Verification items for the finished model (mm, model axes). Face numbers are marked on the shaded views. Coordinates: 2 decimals unless noted, no trailing zeros. Loops run counter-clockwise (first coordinate to the right, second up) from the corner with the lowest first, then second, coordinate; pieces in that order, holes last. Notation, with made-up numbers: (4, -29.75) -> (19, -29.75) arc R28 ccw to (19, 4.25) -> close; hole circle Ø1 at (26, 39). An arc over 180 degrees is marked (long way). Use CSV: the item, a comma, the result in double quotes. Start each with the question number.
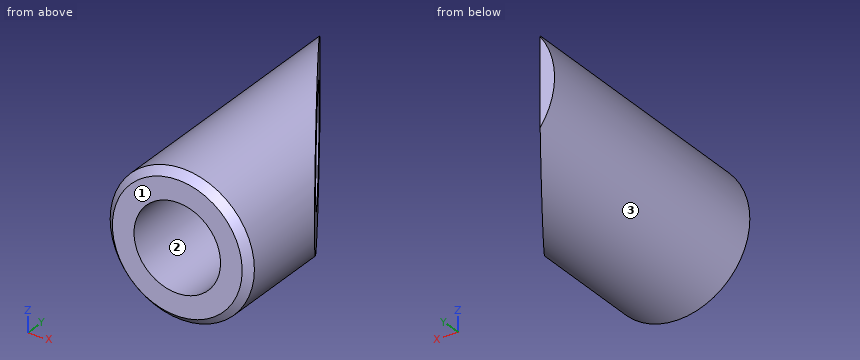
```python
from build123d import *

# Parameters (mm, degrees)
F0_W     = 10
F0_H     = 40
F3_DEPTH = 25
F4_SIZE  = 1
F5_R     = 6
F6_DEPTH = 50


with BuildPart() as f1:
    # F0 (on Top) → F1 (revolve)
    with BuildSketch(Plane.XY):
        with Locations((5, 20)):
            Rectangle(F0_W, F0_H)
    revolve(axis=Axis((0, 20, 0), (0, -1, 0)))

    # F2 (on Top) → F3 (cut, symmetric)
    with BuildSketch(Plane.XY):
        Polygon((10, 40), (-8, 40), (10, 13), align=None)
    extrude(amount=F3_DEPTH, both=True, mode=Mode.SUBTRACT)

    # F4
    f4_edges = [f1.edges().sort_by_distance(p)[0] for p in [
        (-10, 0, 0),
    ]]
    chamfer(f4_edges, length=F4_SIZE)

    # F5 (on face) → F6 (cut)
    with BuildSketch(Plane.XZ):
        Circle(F5_R)
    extrude(amount=-F6_DEPTH, mode=Mode.SUBTRACT)


solid = f1.part
```
1. Scan lines: line 1 (Z direction, x = 0, y = 23.5); line 2 (Z direction, x = -4.5, y = 15.5). Record each from-to range of solid material in increasing order.
2. Depth check by flat-ended pin: pin 1 (3 mm diameter, centred on y = 23, z = 5.5, fed in from -X); pin 2 (6 mm diameter, centred on y = 33, z = 0, fed in from +X); pin 3 (4 mm diameter, centred on y = 21.5, z = 4, fed in from +X). Enter the tip coordinate at first touch or a pass-through.
3. Cross-section at B-B, the plane y = 16. Record the boundary of the cut face in (x, z), plus the area to 3 significant figures.
4. Cross-section at C-C, the plane y = 5. Record the boundary of the cut face in (x, z), plus the area to 3 significant figures.
5. Cross-section at A-A, the plane x = 0. Record the boundary of the cut face in (y, z).
6. Release check for a two-part mould opening along Z. For the marked faces 1, 2 and 3 record: released by +Z, released by -Z, zero draft, split by the parting line, or undercut.
Solution:
1,line 1,"z = -10 to -6, 6 to 10"
1,line 2,"z = -8.93 to -3.97, 3.97 to 8.93"
2,pin 1,"stops at x = -9.17"
2,pin 2,"stops at x = -5.2"
2,pin 3,"stops at x = 5.67"
3,outline,"(8, -6) -> (8, 6) arc R10 ccw (long way) to start; hole circle Ø12 at (0, 0)"
3,area,"185 mm2"
4,outline,"circle Ø20 at (0, 0); hole circle Ø12 at (0, 0)"
4,area,"201 mm2"
5,outline,"(0, -9) -> (1, -10) -> (28, -10) -> (28, -6) -> (0, -6) -> close; (0, 6) -> (28, 6) -> (28, 10) -> (1, 10) -> (0, 9) -> close"
6,face 1,"zero draft"
6,face 2,"undercut"
6,face 3,"split by the parting line"
